from build123d import *

# Parameters (mm, degrees)
SKETCH1_R                     = 2
SKETCH1_R_2                   = 1
BOSS_EXTRUDE1_DEPTH           = 10
SKETCH2_R                     = 1.28905
HOLE_FOR_5_40_SET_SCREW_DEPTH = 3


with BuildPart() as part:
    # Sketch1 → Boss-Extrude1 (new body)
    with BuildSketch(Plane.XY):
        Circle(SKETCH1_R)
        Circle(SKETCH1_R_2, mode=Mode.SUBTRACT)
    extrude(amount=BOSS_EXTRUDE1_DEPTH)

    # Sketch2 → hole for 5-40 set screw (cut, through all)
    with BuildSketch(Plane(origin=(0, 0, 0), x_dir=(0, 0, -1), z_dir=(1, 0, 0))):
        with Locations((-4, 0)):
            Circle(SKETCH2_R)
    extrude(amount=-HOLE_FOR_5_40_SET_SCREW_DEPTH, mode=Mode.SUBTRACT)


solid = part.part
Can you work these out from the model? Positions are in its coordinate system, mm. A direction names the side the tool comes from. Give positions to 0.01 mm unless a question says otherwise; leave off trailing zeros. Order: outer loops, then holes, each group sorted by start corner. A loop starts at its lowest first (then second) coordinate and runs counter-clockwise, first axis right, second up. Notation, with made-up numbers: M -31.5,38 L -18.5,38 A17 cw -18.5,51 Z; hole C 23.25,25 d1. An arc over 180 degrees is marked long. Use one line per item in the form item = value. Start each with the question number.
Item 1: If we section it at D-D (x = -0.15): Write out the boundary of the cut face in (y, z).
Item 2: If we section it at A-A (y = 0): Write out the boundary of the cut face in (x, z).
Item 3: For faces 4 (the cylindrical face through (-0.99, 1.09, 3.31)), 5 (the flat face through (1, -1, 0)), which set-ups out of +Z, -Z, +X, -X, +Y, -Y let a thin tool reach every point of the face, with its end or its side?
Item 4: We'd pull the mould along X, two halves only. Please class faces 1 (the cylindrical face through (1.908, 0.601, 4.93)), 2 (the flat face through (1, -1, 10)), 3 (the cylindrical face through (1, 0, 5)): +X half, -X half, draft (parallel to the pull), parting line (faces both ways), or undercut.
Item 5: If I drill on line 1 along X through (y, z) = (0, 7.75); line 2 along X through (y, z) = (0.75, 6.25), over which ranges is the centre line in solid material (lowest first)?
Item 6: If we section it at C-C (z = 2.25): Write out the boundary of the cut face in (x, y), then the cut area to 3 significant figures.
Item 7: Will these pins go through, and if not, where does the flat tip stop? pin 1 Ø1.2 at (x, y) = (0, 0) entering from -Z; pin 2 Ø2 at (x, z) = (-1.5, 3.5) entering from +Y; pin 3 Ø1.5 at (y, z) = (0, 4) entering from -X; pin 4 Ø1 at (x, y) = (-0.5, 1) entering from -Z.
Item 8: If we section it at B-B (x = -0.8): Write out the boundary of the cut face in (y, z).
Outcome:
q1.outline = M -1.99,0 L -0.99,0 L -0.99,3.17 A1.29 cw -0.99,4.83 L -0.99,10 L -1.99,10 Z; M 0.99,0 L 1.99,0 L 1.99,10 L 0.99,10 L 0.99,4.83 A1.29 cw 0.99,3.17 Z
q2.outline = M -2,0 L -1,0 L -1,2.71 L -2,2.71 Z; M -2,5.29 L -1,5.29 L -1,10 L -2,10 Z; M 1,0 L 2,0 L 2,10 L 1,10 Z
q3.face_4 = -X
q3.face_5 = -Z, +X, -X, +Y, -Y
q4.face_1 = parting line
q4.face_2 = draft
q4.face_3 = undercut
q5.line_1 = -2 to -1, 1 to 2
q5.line_2 = -1.85 to -0.66, 0.66 to 1.85
q6.outline = C 0,0 d4; hole C 0,0 d2
q6.area = 9.42 mm2
q7.pin_1 = through
q7.pin_2 = 1.94
q7.pin_3 = 0.66
q7.pin_4 = 0
q8.outline = M -1.83,0 L -0.6,0 L -0.6,2.86 A1.29 cw -0.6,5.14 L -0.6,10 L -1.83,10 Z; M 0.6,0 L 1.83,0 L 1.83,10 L 0.6,10 L 0.6,5.14 A1.29 cw 0.6,2.86 Z
